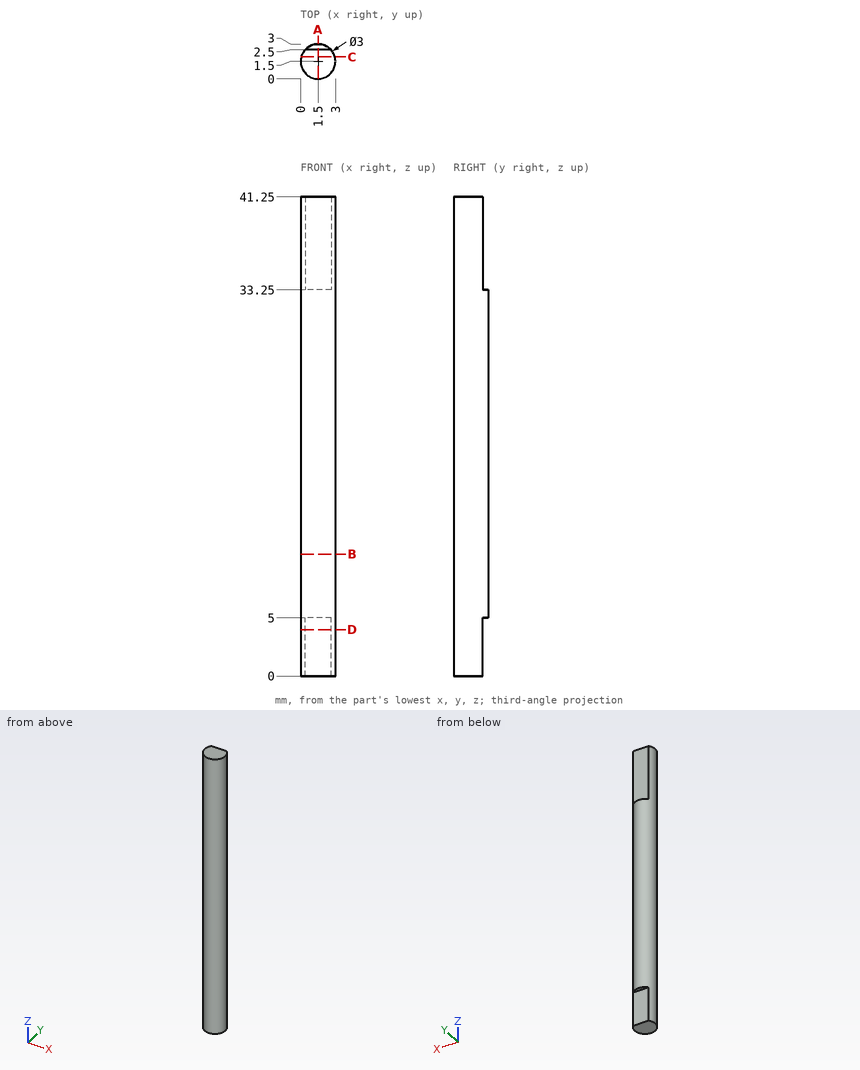
The drawing under review shows one solid part. Ordinate dimensions are in mm from its lowest x, y, z. Round coordinates to 2 decimals unless told otherwise and drop trailing zeros. Loops run counter-clockwise (first coordinate to the right, second up) from the corner with the lowest first, then second, coordinate; pieces in that order, holes last. Notation, with made-up numbers: (19, 35.5) - (34, 35.5) arc R25 cw to (34, 54.5) - close; hole circle Ø5 at (35, -29.5). An arc over 180 degrees is marked (long way). Use a Markdown table: item, result. Add a question column.
Q1. For probe 1 along X at (y, z) = (2.5, 27); probe 2 along Y at (x, z) = (1.4, 18), list the stretches that pass through material, from the lowest coordinate up.
Q2. Add section C-C (y = 1.9). State the section outline as (x, z) points.
Q3. Add section A-A (x = 1.5). State the section outline as (y, z) points, plus the area to 3 significant figures.
Q4. Add section B-B (z = 10.5). State the section outline as (x, y) points, plus the area to 3 significant figures.
Q5. Insertion check: pin 1 Ø1.5 at (y, z) = (1, 22) entering from -X. The pin has a flat end and moves straight along its axis. Give the tip position at first contact, or say it passes through.
Q6. Add section D-D (z = 4). State the section outline as (x, y) points.
Worked answers:
| question | item | result |
|---|---|---|
| 1 | probe 1 | 0.38 to 2.62 |
| 1 | probe 2 | 0 to 3 |
| 2 | outline | (0.05, 0) - (2.95, 0) - (2.95, 41.25) - (0.05, 41.25) - close |
| 3 | outline | (0, 0) - (2.5, 0) - (2.5, 5) - (3, 5) - (3, 33.25) - (2.5, 33.25) - (2.5, 41.25) - (0, 41.25) - close |
| 3 | area | 117 mm² |
| 4 | outline | circle Ø3 at (1.5, 1.5) |
| 4 | area | 7.07 mm² |
| 5 | pin 1 | x = 0 |
| 6 | outline | (0.38, 2.5) arc R1.5 ccw (long way) to (2.62, 2.5) - close |
